```python
from build123d import *

# Parameters (mm, degrees)
BOSS_EXTRUDE1_DEPTH = 60
MOVE_FACE1_DEPTH    = 60
FILLET1_R           = 0.2


# Read off the part's stored shape, not the designer's step: Move Face1
with BuildPart() as part:
    # Sketch1 → Boss-Extrude1 (new body)
    with BuildSketch(Plane(origin=(0, 0, 0), x_dir=(1, 0, 0), z_dir=(0, 1, 0))):
        Polygon((7.721033882, 3.781430367), (3.536999802, -0.218569633), (13.536999802, -0.218569633), (9.721033882, 3.781430367), (18.536999802, 3.781430367), (18.536999802, -1.218569633), (23.536999802, -1.218569633), (23.536999802, 3.781430367), (32.352965722, 3.781430367), (28.536999802, -0.218569633), (38.536999802, -0.218569633), (34.352965722, 3.781430367), (57.036999802, 3.781430367), (57.036999802, -2.218569633), (59.036999802, -2.218569633), (59.036999802, 3.781430367), (59.036999802, 4.781430367), (-16.963000198, 4.781430367), (-16.963000198, 3.781430367), (-16.963000198, -2.218569633), (-14.963000198, -2.218569633), (-14.963000198, 3.781430367), align=None)
    extrude(amount=BOSS_EXTRUDE1_DEPTH)

    # Move Face1 outline → Move Face1 (cut)
    with BuildSketch(Plane(origin=(0, 0, 0), x_dir=(1, 0, 0), z_dir=(0, 1, 0))):
        Polygon((12.836183283, 0.081430367), (4.284936029, 0.081430367), (8.155167552, 3.781430367), (7.721033882, 3.781430367), (3.536999802, -0.218569633), (13.536999802, -0.218569633), (9.721033882, 3.781430367), (9.306414807, 3.781430367), align=None)
        Polygon((-14.963000198, -2.218569633), (-14.963000198, 3.781430367), (-15.263000198, 3.781430367), (-15.263000198, -1.918569633), (-16.663000198, -1.918569633), (-16.663000198, 4.781430367), (-16.963000198, 4.781430367), (-16.963000198, -2.218569633), align=None)
        Polygon((18.836999802, 3.781430367), (18.536999802, 3.781430367), (18.536999802, -1.218569633), (23.536999802, -1.218569633), (23.536999802, 3.781430367), (23.236999802, 3.781430367), (23.236999802, -0.918569633), (18.836999802, -0.918569633), align=None)
        Polygon((59.036999802, 4.781430367), (58.736999802, 4.781430367), (58.736999802, -1.918569633), (57.336999802, -1.918569633), (57.336999802, 3.781430367), (57.036999802, 3.781430367), (57.036999802, -2.218569633), (59.036999802, -2.218569633), align=None)
        Polygon((32.767584796, 3.781430367), (32.352965722, 3.781430367), (28.536999802, -0.218569633), (38.536999802, -0.218569633), (34.352965722, 3.781430367), (33.918832051, 3.781430367), (37.789063575, 0.081430367), (29.23781632, 0.081430367), align=None)
    extrude(amount=MOVE_FACE1_DEPTH, mode=Mode.SUBTRACT)

    # Fillet1
    fillet1_edges = [part.edges().sort_by_distance(p)[0] for p in [
        (-15.263000198, 30, 1.918569633),
        (-16.663000198, 30, 1.918569633),
        (58.736999802, 30, 1.918569633),
        (57.336999802, 30, 1.918569633),
        (33.918832051, 30, -3.781430367),
        (37.789063575, 30, -0.081430367),
        (29.23781632, 30, -0.081430367),
        (32.767584796, 30, -3.781430367),
        (23.236999802, 30, 0.918569633),
        (18.836999802, 30, 0.918569633),
        (9.306414807, 30, -3.781430367),
        (12.836183283, 30, -0.081430367),
        (4.284936029, 30, -0.081430367),
        (8.155167552, 30, -3.781430367),
    ]]
    fillet(fillet1_edges, radius=FILLET1_R)


solid = part.part
```
Input: part model. Units: mm. Frame: model coordinates. A direction names the side the tool comes from. Coordinates: 2 decimals unless noted, no trailing zeros. Write each loop counter-clockwise with the first axis right and the second up, starting at its lowest first coordinate (ties: lowest second). Pieces come first, ordered by that corner, then holes. Notation, with made-up numbers: (39, 59) - (96, 59) arc R29 ccw to (96, 85) - close; hole circle Ø11 at (22, -39.5). An arc over 180 degrees is marked (long way). Put each result on its own line as item: value. Start each with the question number.
1) Cut plane D-D (x = 21). Return the cut outline in (y, z).
2) Reachability of faces 1 (the face through (57.337, 30, -1)), 2 (the face through (30.98, 29.58, -1.91)), 3 (the face through (58.737, 30, -2)) from +Z, -Z, +X, -X, +Y, -Y: full face, straight path, thin tool, end or side. Return the list, or none.
3) Cut plane A-A (z = -2.25). Return the cut outline in (x, y), plus the area to 3 significant figures.
4) Contact query for flat-ended pins moving along their axis: pin 1 (7 mm diameter, centred on x = 44, y = 43.5, fed in from +Z); pin 2 (8.5 mm diameter, centred on x = 9.5, y = 36.5, fed in from +Z); pin 3 (2 mm diameter, centred on x = 20.5, y = 39, fed in from +Z). Output: stop coordinate, or through.
5) Cut plane C-C (x = -4.5). Return the cut outline in (y, z).
6) Ray query, L1, parallel to X at y = 46, z = 0.75; L2, parallel to X at y = 20.5, z = 1.25; L3, parallel to X at y = 11.5, z = -3.25. Return the intervals inside material, ascending.
Resolved:
1. outline: (0, -4.78) - (60, -4.78) - (60, 0.92) - (0, 0.92) - close
2. face 1: +Z, +Y, -Y
2. face 2: +Y, -Y
2. face 3: +Z, -Z, +X, +Y, -Y
3. outline: (-16.66, 0) - (-15.26, 0) - (-15.26, 60) - (-16.66, 60) - close; (6.55, 0) - (10.77, 0) - (10.77, 60) - (6.55, 60) - close; (18.84, 0) - (23.24, 0) - (23.24, 60) - (18.84, 60) - close; (31.31, 0) - (35.52, 0) - (35.52, 60) - (31.31, 60) - close; (57.34, 0) - (58.74, 0) - (58.74, 60) - (57.34, 60) - close
3. area: 938 mm2
4. pin 1: stops at z = -3.78
4. pin 2: stops at z = -0.08
4. pin 3: stops at z = 0.92
5. outline: (0, -4.78) - (60, -4.78) - (60, -3.78) - (0, -3.78) - close
6. L1: x = -16.66 to -15.26, 18.84 to 23.23, 57.34 to 58.74
6. L2: x = -16.66 to -15.26, 57.34 to 58.74
6. L3: x = -16.66 to -15.26, 7.6 to 9.81, 18.84 to 23.24, 32.26 to 34.47, 57.34 to 58.74
